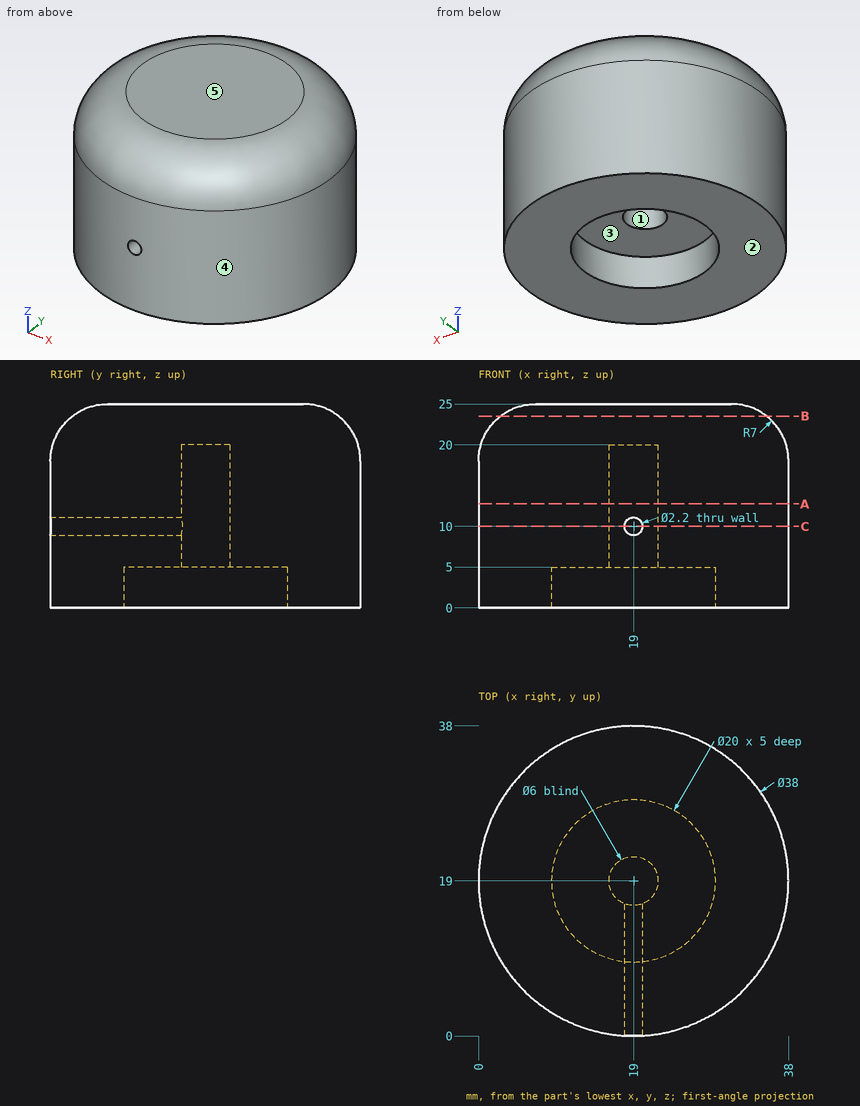
For this review, use the dimensioned drawing (mm, ordinates from the lowest corner) and the shaded views. A direction names the side the tool comes from. Round coordinates to 2 decimals unless told otherwise and drop trailing zeros. Order: outer loops, then holes, each group sorted by start corner. A loop starts at its lowest first (then second) coordinate and runs counter-clockwise, first axis right, second up. Notation, with made-up numbers: M 17,-26 L 23,-26 A11 ccw 23,-14 Z; hole C 80,42 d10. An arc over 180 degrees is marked long. Write each question's results on one line, items separated by ' | '. Start each with the question number.
1. Add section B-B (z = 23.5). State the section outline as (x, y) points.
2. Draft analysis for pull direction X (two halves, no side actions). For the marked faces 3, 4 and 5, state which applies: pulls with the +X half, pulls with the -X half, needs draft (parallel to the pull), parting line crosses it, or undercut.
3. Clearance check with flat-ended pins moving along their axes: pin 1 Ø5 at (x, y) = (25.5, 18) entering from -Z; pin 2 Ø1 at (x, z) = (22, 4) entering from -Y; pin 3 Ø4 at (x, z) = (26.5, 16) entering from +Y. State where each tip first meets the part, or that it passes through.
4. Add section C-C (z = 10). State the section outline as (x, y) points.
5. To check wall thickness, follow L1, parallel to Y at x = 19, z = 3.9; L2, parallel to Y at x = 19, z = 10.75; L3, parallel to Z at x = 14, y = 11. State the ranges of each line that lie inside material, in increasing order. Write a range as [from, to].
6. Add section A-A (z = 12.75). State the section outline as (x, y) points.
7. Tool access review of the marked faces 1 and 2: name each direction out of +Z, -Z, +X, -X, +Y, -Y from which nothing blocks a thin tool from reaching the whole face with its end or side.
Output values:
1) outline: C 19,19 d32.66
2) face 3: undercut | face 4: parting line crosses it | face 5: needs draft
3) pin 1: z = 5 | pin 2: y = 0.17 | pin 3: y = 37.19
4) outline: M 17.9,0.03 L 17.9,16.21 A3 cw long 20.1,16.21 L 20.1,0.03 A19 ccw long Z
5) L1: [0, 9], [29, 38] | L2: [22, 38] | L3: [5, 25]
6) outline: C 19,19 d38; hole C 19,19 d6
7) face 1: -Z | face 2: -Z, +X, -X, +Y, -Y
